```python
from build123d import *

# Parameters (mm, degrees)
F0_W     = 100
F0_H     = 90
F1_DEPTH = 70
F2_W     = 60
F2_H     = 70
F3_DEPTH = 100.001
F4_W     = 40
F4_H     = 50
F5_DEPTH = 20.001
F6_R     = 7
F7_DEPTH = 20.001


with BuildPart() as f1:
    # F0 (on Front) → F1 (new body)
    with BuildSketch(Plane.XZ):
        with Locations((-20, -25)):
            Rectangle(F0_W, F0_H)
    extrude(amount=F1_DEPTH)

    # F2 (on face) → F3 (cut, through all)
    with BuildSketch(Plane.YZ.offset(30)):
        with Locations((-50, -5)):
            Rectangle(F2_W, F2_H)
    extrude(amount=-F3_DEPTH, mode=Mode.SUBTRACT)

    # F4 (on face) → F5 (cut, through all)
    with BuildSketch(Plane.XZ.offset(20)):
        with Locations((-60, 5)):
            Rectangle(F4_W, F4_H)
    extrude(amount=-F5_DEPTH, mode=Mode.SUBTRACT)

    # F6 (on face) → F7 (cut, through all)
    with BuildSketch(Plane.XZ.offset(20)):
        Circle(F6_R)
    extrude(amount=-F7_DEPTH, mode=Mode.SUBTRACT)


solid = f1.part
```
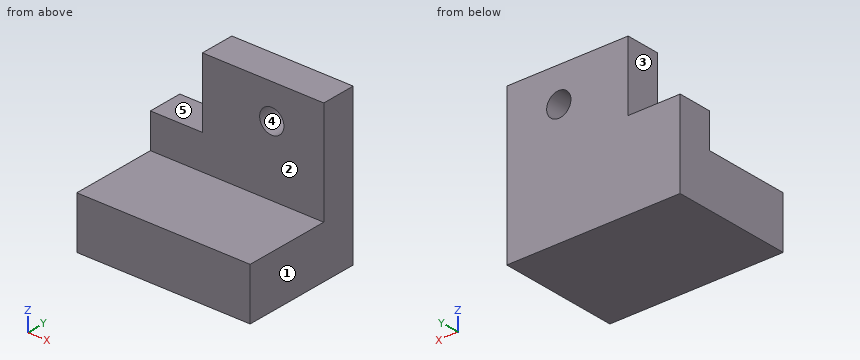
Source: CAD feature listing. Evaluate the final solid. Frame: model axes, mm. Face numbers are marked on the shaded views. A direction names the side the tool comes from. Give positions to 0.01 mm unless a question says otherwise; leave off trailing zeros. Order: outer loops, then holes, each group sorted by start corner. A loop starts at its lowest first (then second) coordinate and runs counter-clockwise, first axis right, second up.
(1) Section query A-A (z = 0). Return the cut outline in (x, y), plus the area to 3 significant figures.
(2) Material intervals for line 1 along Z through (x, y) = (0, -9); line 2 along X through (y, z) = (-17.5, 10); line 3 along Y through (x, z) = (20.5, 10), sorted ascending.
(3) Contact query for flat-ended pins moving along their axis: P1, Ø8.5, axis at x = 0, z = 0, coming from the +Y side; P2, Ø10, axis at x = 8, y = -51.5, coming from the +Z side; P3, Ø22, axis at y = -15, z = 8.5, coming from the -X side. Output: stop coordinate, or through.
(4) Section query C-C (y = -8). Return the cut outline in (x, z), plus the area to 3 significant figures.
(5) Section query B-B (x = 0). Return the cut outline in (y, z), plus the area to 3 significant figures.
(6) Section query D-D (x = -20). Return the cut outline in (y, z).
(7) Access query for the marked faces 1 and 2. Directions: +Z, -Z, +X, -X, +Y, -Y. A direction counts if a zero-diameter tool reaches every point of the face in a straight line with its end or side. Return the directions, or none.
(8) Pull-direction query (Z, two-part tool) for the marked faces 3, 4 and 5; classes: +Z half, -Z half, draft (parallel to the pull), parting line (faces both ways), or undercut.
Outcome:
1. outline: (-40, -20) - (-7, -20) - (-7, 0) - (-40, 0) - close; (7, -20) - (30, -20) - (30, 0) - (7, 0) - close
1. area: 1,120 mm2
2. line 1: z = -70 to -7, 7 to 20
2. line 2: x = -40 to 30
2. line 3: y = -20 to 0
3. P1: passes through
3. P2: stops at z = -40
3. P3: stops at x = -40
4. outline: (-70, -70) - (30, -70) - (30, 20) - (-40, 20) - (-40, -20) - (-70, -20) - close; hole circle Ø14 at (0, 0)
4. area: 7,650 mm2
5. outline: (-70, -70) - (0, -70) - (0, -7) - (-20, -7) - (-20, -40) - (-70, -40) - close; (-20, 7) - (0, 7) - (0, 20) - (-20, 20) - close
5. area: 3,020 mm2
6. outline: (-70, -70) - (0, -70) - (0, 20) - (-20, 20) - (-20, -40) - (-70, -40) - close
7. face 1: +Z, -Z, +X, +Y, -Y
7. face 2: +Z, +X, -X, -Y
8. face 3: draft
8. face 4: undercut
8. face 5: +Z half
